Here's how the part is built. I have some questions about the finished solid (model axes, mm). A direction names the side the tool comes from. Round coordinates to 2 decimals unless told otherwise and drop trailing zeros. Write each loop counter-clockwise with the first axis right and the second up, starting at its lowest first coordinate (ties: lowest second). Pieces come first, ordered by that corner, then holes. Notation, with made-up numbers: (69.25, -29.5) - (120.25, -29.5) arc R13 ccw to (120.25, -23.5) - close; hole circle Ø10 at (-2, 71). An arc over 180 degrees is marked (long way). One line per question, with ' | ' between items. Start each with the question number.
(1) Imagine slicing it at A-A (y = -150.5). Write out the boundary of the cut face in (x, z), plus the area to 3 significant figures.
(2) For faces 4 (the flat face through (154.1, -109.3, 1.5)), 5 (the flat face through (143, -105, 0)), which set-ups out of +Z, -Z, +X, -X, +Y, -Y let a thin tool reach every point of the face, with its end or its side?
(3) Will these pins go through, and if not, where does the flat tip stop? pin 1 (1.5 mm diameter, centred on y = -188, z = 1, fed in from -X); pin 2 (8 mm diameter, centred on x = 35.5, y = -70, fed in from +Z); pin 3 (1.5 mm diameter, centred on x = 84.5, z = 2, fed in from -Y).
(4) Thinking about a two-plate mould opening in Y: for faces 1 (the flat face through (59.434, -108.95, 1.521)), 2 (the flat face through (168.507, -108.95, 1.521)), 3 (the flat face through (143, -105, 3)), which applies, pulls with the +Y half, pulls with the -Y half, needs draft (parallel to the pull), parting line crosses it, or undercut?
(5) Imagine slicing it at C-C (x = 128.5). Write out the boundary of the cut face in (y, z), plus the area to 3 significant figures.
(6) Imagine slicing it at D-D (z = 1.05). Give the number of separate pieces and of enclosed holes in the cut face, plus the area to 3 significant figures.
(7) If I drill on L1, parallel to Y at x = 176, z = 1.7; L2, parallel to X at y = -82.5, z = 1.15; L3, parallel to X at y = -154, z = 1.15, over which ranges is the centre line in solid material (lowest first)?
(8) Imagine slicing it at B-B (x = 71.5). Write out the boundary of the cut face in (y, z), plus the area to 3 significant figures.
Autodesk Inventor part; units mm, degrees
ref_plane "YZ Plane" through (0, 0, 0) normal (1, 0, 0) x (0, 1, 0)
ref_plane "XZ Plane" through (0, 0, 0) normal (0, 1, 0) x (-1, 0, 0)
ref_plane "XY Plane" through (0, 0, 0) normal (0, 0, 1) x (1, 0, 0)
sketch "草圖1" plane through (0, 0, 0) normal (0, 0, 1) x (1, 0, 0)
  line L0 (0, 0) -> (290, 0)
  line L1 (290, 0) -> (290, -195)
  line L2 (290, -195) -> (0, -195)
  line L3 (0, -195) -> (0, 0)
  line L4 (15, -59.78) -> (23, -59.78)
  line L5 (23, -59.78) -> (23, -62.73)
  line L6 (23, -62.73) -> (15, -62.73)
  line L7 (15, -62.73) -> (15, -59.78)
  line L8 (15, -81.65) -> (23, -81.65)
  line L9 (23, -81.65) -> (23, -84.6)
  line L10 (23, -84.6) -> (15, -84.6)
  line L11 (15, -84.6) -> (15, -81.65)
  line L12 (15, -133.65) -> (23, -133.65)
  line L13 (23, -133.65) -> (23, -136.6)
  line L14 (23, -136.6) -> (15, -136.6)
  line L15 (15, -136.6) -> (15, -133.65)
  line L16 (15, -158.57) -> (23, -158.57)
  line L17 (23, -158.57) -> (23, -161.52)
  line L18 (23, -161.52) -> (15, -161.52)
  line L19 (15, -161.52) -> (15, -158.57)
  line L20 (275, -81.65) -> (275, -84.6)
  line L21 (275, -59.78) -> (275, -62.73)
  line L22 (267, -81.65) -> (275, -81.65)
  line L23 (275, -62.73) -> (267, -62.73)
  line L24 (267, -59.78) -> (275, -59.78)
  line L25 (275, -84.6) -> (267, -84.6)
  line L26 (267, -84.6) -> (267, -81.65)
  line L27 (267, -62.73) -> (267, -59.78)
  line L28 (267, -133.65) -> (275, -133.65)
  line L29 (275, -133.65) -> (275, -136.6)
  line L30 (267, -136.6) -> (267, -133.65)
  line L31 (275, -136.6) -> (267, -136.6)
  line L32 (267, -158.57) -> (275, -158.57)
  line L33 (275, -158.57) -> (275, -161.52)
  line L34 (275, -161.52) -> (267, -161.52)
  line L35 (267, -161.52) -> (267, -158.57)
  line L36 (0, -97.5) -> (290, -97.5) construction
  line L37 (19, -84.6) -> (19, -133.65) construction
  line L38 (145, 0) -> (145, -195) construction
  line L39 (23, -83.125) -> (267, -83.125) construction
  point P0 (15, -83.125)
  point P1 (15, -61.255)
  point P2 (15, -135.125)
  point P3 (15, -160.045)
  point P4 (267, -61.255)
  point P5 (267, -135.125)
  point P6 (267, -160.045)
  point P7 (145, -83.125)
  dimension "d0" = 2.95
  dimension "d1" = 8
  dimension "d3" = 52
  dimension "d5" = 195
  dimension "d6" = 290
  dimension "d9" = 252
  dimension "d16" = 12.9
  dimension "d36" = 18.92
  dimension "d37" = 21.97
extrude "擠出1" add sketch "草圖1" along normal blind 3
sketch "草圖3" plane through (0, 0, 3) normal (0, 0, 1) x (1, 0, 0)
  line L0 (290, 0) -> (0, 0)
  line L1 (0, 0) -> (290, 0)
  line L2 (290, 0) -> (290, -50)
  line L3 (290, -50) -> (0, -50)
  line L4 (0, -50) -> (0, 0)
  line L5 (290, -195) -> (290, 0)
  line L6 (42.05, -195) -> (45, -195)
  line L7 (45, -195) -> (45, -180)
  line L8 (45, -180) -> (42.05, -180)
  line L9 (42.05, -180) -> (42.05, -195)
  line L10 (0, -195) -> (290, -195)
  line L11 (245, -195) -> (247.95, -195)
  line L12 (247.95, -195) -> (247.95, -180)
  line L13 (247.95, -180) -> (245, -180)
  line L14 (245, -180) -> (245, -195)
  line L15 (45, -187.5) -> (245, -187.5)
  point P0 (145, -195)
  point P1 (145, -187.5)
  point P2 (247.95, -195)
  dimension "d17" = 50
  dimension "d18" = 200
  dimension "d19" = 2.95
  dimension "d20" = 2.95
  dimension "d22" = 15
  dimension "d23" = 0
extrude "擠出2" cut sketch "草圖3" against normal up to surface (3 mm away) contours L2 L3 L4 L0 | L10 L14 L13 L12 | L6 L9 L8 L7
sketch "草圖6" plane through (0, 0, 3) normal (0, 0, 1) x (1, 0, 0)
  line L0 (6, -136.6) -> (284, -136.6)
  line L1 (284, -136.6) -> (284, -158.57)
  line L2 (284, -158.57) -> (6, -158.57)
  line L3 (6, -158.57) -> (6, -136.6)
  line L4 (23, -136.6) -> (15, -136.6)
  line L5 (15, -158.57) -> (23, -158.57)
  line L6 (0, -50) -> (0, -195)
  line L7 (290, -195) -> (290, -50)
  line L8 (6, -81.65) -> (6, -62.73)
  line L9 (6, -62.73) -> (284, -62.73)
  line L10 (284, -62.73) -> (284, -81.65)
  line L11 (284, -81.65) -> (6, -81.65)
  line L12 (15, -81.65) -> (23, -81.65)
  line L13 (23, -62.73) -> (15, -62.73)
  line L14 (20.4049, -96.65) -> (34.8098, -121.6)
  line L15 (34.8098, -121.6) -> (6, -121.6)
  line L16 (6, -121.6) -> (20.4049, -96.65)
  line L17 (37.7254, -96.65) -> (66.5352, -96.65)
  line L18 (66.5352, -96.65) -> (52.1303, -121.6)
  line L19 (52.1303, -121.6) -> (37.7254, -96.65)
  line L20 (105.3098, -121.6) -> (76.5, -121.6)
  line L21 (76.5, -121.6) -> (90.9049, -96.65)
  line L22 (90.9049, -96.65) -> (105.3098, -121.6)
  line L23 (122.6303, -121.6) -> (108.2254, -96.65)
  line L24 (137.0352, -96.65) -> (122.6303, -121.6)
  line L25 (108.2254, -96.65) -> (137.0352, -96.65)
  line L26 (175.8098, -121.6) -> (147, -121.6)
  line L27 (147, -121.6) -> (161.4049, -96.65)
  line L28 (161.4049, -96.65) -> (175.8098, -121.6)
  line L29 (193.1303, -121.6) -> (178.7254, -96.65)
  line L30 (207.5352, -96.65) -> (193.1303, -121.6)
  line L31 (178.7254, -96.65) -> (207.5352, -96.65)
  line L32 (246.3098, -121.6) -> (217.5, -121.6)
  line L33 (217.5, -121.6) -> (231.9049, -96.65)
  line L34 (231.9049, -96.65) -> (246.3098, -121.6)
  line L35 (263.6303, -121.6) -> (249.2254, -96.65)
  line L36 (278.0352, -96.65) -> (263.6303, -121.6)
  line L37 (249.2254, -96.65) -> (278.0352, -96.65)
  line L38 (45, -195) -> (245, -195)
  line L39 (60, -195) -> (230, -195)
  line L40 (230, -195) -> (230, -175)
  line L41 (230, -175) -> (60, -175)
  line L42 (60, -175) -> (60, -195)
  line L43 (262.95, -195) -> (290, -195)
  line L44 (290, -195) -> (290, -175)
  line L45 (290, -175) -> (262.95, -175)
  line L46 (262.95, -175) -> (262.95, -195)
  line L47 (0, -195) -> (42.05, -195)
  line L48 (27.05, -195) -> (0, -195)
  line L49 (0, -195) -> (0, -175)
  line L50 (0, -175) -> (27.05, -175)
  line L51 (27.05, -175) -> (27.05, -195)
  line L52 (42.05, -195) -> (42.05, -180)
  line L53 (45, -180) -> (45, -195)
  line L54 (245, -195) -> (245, -180)
  line L55 (247.95, -180) -> (247.95, -195)
  point P0 (0, 0)
  point P1 (284, -147.585)
  point P2 (20.4049, -113.2833)
  point P3 (52.1303, -104.9667)
  point P4 (122.6303, -104.9667)
  point P5 (90.9049, -113.2833)
  point P6 (193.1303, -104.9667)
  point P7 (161.4049, -113.2833)
  point P8 (263.6303, -104.9667)
  point P9 (231.9049, -113.2833)
  point P10 (42.05, -187.5)
  dimension "d32" = 6
  dimension "d33" = 6
  dimension "d39" = 15
  dimension "d40" = 15
  dimension "d41" = 15
  dimension "d44" = 70.5
  dimension "d49" = 20
  dimension "d50" = 15
  dimension "d51" = 15
  dimension "d52" = 15
  dimension "d53" = 15
extrude "擠出5" cut sketch "草圖6" against normal up to surface (3 mm away)
sketch "草圖8" plane through (0, 0, 3) normal (0, 0, 1) x (1, 0, 0)
  line L0 (275, -62.73) -> (284, -62.73)
  line L1 (284, -62.73) -> (284, -81.65)
  line L2 (284, -81.65) -> (275, -81.65)
  line L3 (275, -81.65) -> (275, -84.6)
  line L4 (275, -84.6) -> (267, -84.6)
  line L5 (267, -84.6) -> (267, -81.65)
  line L6 (267, -81.65) -> (23, -81.65)
  line L7 (23, -81.65) -> (23, -84.6)
  line L8 (23, -84.6) -> (15, -84.6)
  line L9 (15, -84.6) -> (15, -81.65)
  line L10 (15, -81.65) -> (6, -81.65)
  line L11 (6, -81.65) -> (6, -62.73)
  line L12 (6, -62.73) -> (15, -62.73)
  line L13 (15, -62.73) -> (15, -59.78)
  line L14 (15, -59.78) -> (23, -59.78)
  line L15 (23, -59.78) -> (23, -62.73)
  line L16 (23, -62.73) -> (267, -62.73)
  line L17 (267, -62.73) -> (267, -59.78)
  line L18 (267, -59.78) -> (275, -59.78)
  line L19 (275, -59.78) -> (275, -62.73)
  line L20 (15, -158.57) -> (6, -158.57)
  line L21 (6, -158.57) -> (6, -136.6)
  line L22 (6, -136.6) -> (15, -136.6)
  line L23 (15, -136.6) -> (15, -133.65)
  line L24 (15, -133.65) -> (23, -133.65)
  line L25 (23, -133.65) -> (23, -136.6)
  line L26 (23, -136.6) -> (267, -136.6)
  line L27 (267, -136.6) -> (267, -133.65)
  line L28 (267, -133.65) -> (275, -133.65)
  line L29 (275, -133.65) -> (275, -136.6)
  line L30 (275, -136.6) -> (284, -136.6)
  line L31 (284, -136.6) -> (284, -158.57)
  line L32 (284, -158.57) -> (275, -158.57)
  line L33 (275, -158.57) -> (275, -161.52)
  line L34 (275, -161.52) -> (267, -161.52)
  line L35 (267, -161.52) -> (267, -158.57)
  line L36 (267, -158.57) -> (23, -158.57)
  line L37 (23, -158.57) -> (23, -161.52)
  line L38 (23, -161.52) -> (15, -161.52)
  line L39 (15, -161.52) -> (15, -158.57)
  line L40 (52.1303, -121.6) -> (37.7254, -96.65)
  line L41 (37.7254, -96.65) -> (66.5352, -96.65)
  line L42 (66.5352, -96.65) -> (52.1303, -121.6)
  line L43 (207.5352, -96.65) -> (193.1303, -121.6)
  line L44 (193.1303, -121.6) -> (178.7254, -96.65)
  line L45 (178.7254, -96.65) -> (207.5352, -96.65)
  line L46 (108.2254, -96.65) -> (137.0352, -96.65)
  line L47 (137.0352, -96.65) -> (122.6303, -121.6)
  line L48 (122.6303, -121.6) -> (108.2254, -96.65)
  line L49 (249.2254, -96.65) -> (278.0352, -96.65)
  line L50 (278.0352, -96.65) -> (263.6303, -121.6)
  line L51 (263.6303, -121.6) -> (249.2254, -96.65)
  line L52 (90.9049, -96.65) -> (105.3098, -121.6)
  line L53 (105.3098, -121.6) -> (76.5, -121.6)
  line L54 (76.5, -121.6) -> (90.9049, -96.65)
  line L55 (147, -121.6) -> (161.4049, -96.65)
  line L56 (161.4049, -96.65) -> (175.8098, -121.6)
  line L57 (175.8098, -121.6) -> (147, -121.6)
  line L58 (34.8098, -121.6) -> (6, -121.6)
  line L59 (6, -121.6) -> (20.4049, -96.65)
  line L60 (20.4049, -96.65) -> (34.8098, -121.6)
  line L61 (217.5, -121.6) -> (231.9049, -96.65)
  line L62 (231.9049, -96.65) -> (246.3098, -121.6)
  line L63 (246.3098, -121.6) -> (217.5, -121.6)
  line L64 (262.95, -195) -> (262.95, -175)
  line L65 (262.95, -175) -> (290, -175)
  line L66 (290, -175) -> (290, -50)
  line L67 (290, -50) -> (0, -50)
  line L68 (0, -50) -> (0, -175)
  line L69 (0, -175) -> (27.05, -175)
  line L70 (27.05, -175) -> (27.05, -195)
  line L71 (27.05, -195) -> (42.05, -195)
  line L72 (42.05, -195) -> (42.05, -180)
  line L73 (42.05, -180) -> (45, -180)
  line L74 (45, -180) -> (45, -195)
  line L75 (45, -195) -> (60, -195)
  line L76 (60, -195) -> (60, -175)
  line L77 (60, -175) -> (230, -175)
  line L78 (230, -175) -> (230, -195)
  line L79 (230, -195) -> (245, -195)
  line L80 (245, -195) -> (245, -180)
  line L81 (245, -180) -> (247.95, -180)
  line L82 (247.95, -180) -> (247.95, -195)
  line L83 (247.95, -195) -> (262.95, -195)
  point P0 (0, 0)
Check sheet entries:
1) outline: (0, 0) - (6, 0) - (6, 3) - (0, 3) - close; (284, 0) - (290, 0) - (290, 3) - (284, 3) - close | area: 36.0 mm^2
2) face 4: +Z, -Z | face 5: -Z, +X, -X, +Y, -Y
3) pin 1: x = 27.05 | pin 2: through | pin 3: y = -175
4) face 1: undercut | face 2: undercut | face 3: needs draft
5) outline: (-175, 0) - (-158.57, 0) - (-158.57, 3) - (-175, 3) - close; (-136.6, 0) - (-111.43, 0) - (-111.43, 3) - (-136.6, 3) - close; (-96.65, 0) - (-81.65, 0) - (-81.65, 3) - (-96.65, 3) - close; (-62.73, 0) - (-50, 0) - (-50, 3) - (-62.73, 3) - close | area: 208 mm^2
6) separate pieces: 1 | enclosed holes: 10 | area: 23,000 mm^2
7) L1: -175 to -158.57, -136.6 to -81.65, -62.73 to -50 | L2: 0 to 15, 23 to 267, 275 to 290 | L3: 0 to 6, 284 to 290
8) outline: (-175, 0) - (-158.57, 0) - (-158.57, 3) - (-175, 3) - close; (-136.6, 0) - (-81.65, 0) - (-81.65, 3) - (-136.6, 3) - close; (-62.73, 0) - (-50, 0) - (-50, 3) - (-62.73, 3) - close | area: 252 mm^2
